Could you check a few things on this model? Use its own coordinates, in mm. A direction names the side the tool comes from. Round coordinates to 2 decimals unless told otherwise and drop trailing zeros. Loops run counter-clockwise (first coordinate to the right, second up) from the corner with the lowest first, then second, coordinate; pieces in that order, holes last. Notation, with made-up numbers: (-5.5, 73) -> (28.5, 73) arc R12 ccw to (28.5, 83) -> close; hole circle Ø5 at (-33.5, 20). An arc over 180 degrees is marked (long way). Put each result on its own line as item: value. Start each with the question number.
1. I need wall thicknesses on line 1 (Y direction, x = 0.75, z = -17); line 2 (Z direction, x = 2.35, y = 11.95); line 3 (Y direction, x = 1.6, z = -8). Which ranges of each line are inside material? Lowest first, please. Write a range as [from, to].
2. Imagine slicing it at A-A, the plane y = 25.81. Please give me the cut outline in (x, z).
3. I'm going to push a flat-ended pin straight in: P1, Ø1.5, axis at x = 1, y = 62, coming from the +Z side. Where does the tip first touch, or does it pass through?
4. Which directions (+Z, -Z, +X, -X, +Y, -Y) give clear straight access to the entire face, cutting with the end or side of a thin tool? Please do faces 1 (the cylindrical face through (2, 22, -31)), 2 (the flat face through (2, 12, -29.15)), 3 (the flat face through (2, 55, -2)).
5. If we mould it in two halves opening along Y, with no side actions, what happens to faces 4 (the flat face through (2, 49, -22)), 5 (the cylindrical face through (1.57, 65.92, -7.36)), 6 (the cylindrical face through (1.568, 43.931, -8.462)), 7 (the cylindrical face through (1.612, 39.854, -1.765))? For each: pulls with the +Y half, pulls with the -Y half, needs draft (parallel to the pull), parting line crosses it, or undercut.
6. Imagine slicing it at D-D, the plane x = 2.1. Count the separate pieces of the cut face and the enclosed holes in it, and give its area (3 significant figures).
7. Imagine slicing it at B-B, the plane z = -7. Please give me the cut outline in (x, y) (3 decimals), and give its area (3 significant figures).
8. Imagine slicing it at C-C, the plane y = 7. Please give me the cut outline in (x, z), and give its area (3 significant figures).
```python
from build123d import *

# Parameters (mm, degrees)
SKETCH1_R             = 5.075
SKETCH1_R_2           = 1.65
SKETCH1_R_3           = 2.1
SKETCH1_R_4           = 0.8
SKETCH1_W             = 13
SKETCH1_H             = 18
BOSS_EXTRUDE1_DEPTH   = 3.18
SKETCH3_R             = 5.5
CUT_EXTRUDE4_DEPTH    = 78.831812262
FILLET2_R             = 3
CHAMFER2_SIZE         = 1.8
FILLET4_R             = 0.5
M2_TAPPED_HOLE1_D     = 1.6
FILLET9_R             = 1
FILLET11_R            = 5
M3X0_5_TAPPED_HOLE1_D = 2.5


with BuildPart() as part:
    # Sketch1 → Boss-Extrude1 (new body)
    with BuildSketch(Plane(origin=(0, 0, 0), x_dir=(0, 0, -1), z_dir=(1, 0, 0))):
        Polygon((0, 0), (0, 37.775), (2, 39.775), (2, 70.81), (22, 70.81), (22, 23.81), (32.15, 23.81), (32.15, 0), align=None)
        with Locations(Location((7, 32.7, 0), (0, 0, 180))):
            Circle(SKETCH1_R, mode=Mode.SUBTRACT)
        with Locations(Location((7, 64.31, 0), (0, 0, 180))):
            Circle(SKETCH1_R_2, mode=Mode.SUBTRACT)
        with Locations(Location((17, 62.31, 0), (0, 0, 180))):
            Circle(SKETCH1_R_2, mode=Mode.SUBTRACT)
        with Locations(Location((3.15, 5.95, 0), (0, 0, 180))):
            Circle(SKETCH1_R_3, mode=Mode.SUBTRACT)
        with Locations(Location((3.15, 11.95, 0), (0, 0, 180))):
            Circle(SKETCH1_R_3, mode=Mode.SUBTRACT)
        with Locations(Location((10.15, 4.95, 0), (0, 0, 180))):
            Circle(SKETCH1_R_4, mode=Mode.SUBTRACT)
        with Locations(Location((3.15, 16.95, 0), (0, 0, 180))):
            Circle(SKETCH1_R_4, mode=Mode.SUBTRACT)
        with Locations((22.65, 11.81)):
            Rectangle(SKETCH1_W, SKETCH1_H, mode=Mode.SUBTRACT)
    extrude(amount=BOSS_EXTRUDE1_DEPTH)

    # Sketch3 → Cut-Extrude4 (cut, through all)
    with BuildSketch(Plane.ZY):
        with Locations((-11, 48.810865899)):
            Circle(SKETCH3_R)
    extrude(amount=-CUT_EXTRUDE4_DEPTH, mode=Mode.SUBTRACT)

    # Fillet2
    fillet2_edges = [part.edges().sort_by_distance(p)[0] for p in [
        (1.59, 0, 0),
        (1.59, 37.775, 0),
        (1.59, 39.775, -2),
    ]]
    fillet(fillet2_edges, radius=FILLET2_R)

    # Chamfer2
    chamfer2_edges = [part.edges().sort_by_distance(p)[0] for p in [
        (1.59, 70.81, -2),
        (1.59, 70.81, -22),
    ]]
    chamfer(chamfer2_edges, length=CHAMFER2_SIZE)

    # Fillet4
    fillet4_edges = [part.edges().sort_by_distance(p)[0] for p in [
        (1.59, 69.01, -22),
        (1.59, 69.01, -2),
    ]]
    fillet(fillet4_edges, radius=FILLET4_R)

    # M2 Tapped Hole1 (through all)
    with Locations(Plane(origin=(0, 16.95, -3.15), x_dir=(0, 0, -1), z_dir=(-1, 0, 0))):
        with Locations((0, 0), (7, 12)):
            Hole(M2_TAPPED_HOLE1_D / 2)

    # Fillet9
    fillet9_edges = [part.edges().sort_by_distance(p)[0] for p in [
        (1.59, 20.81, -16.15),
        (1.59, 2.81, -16.15),
        (1.59, 2.81, -29.15),
        (1.59, 20.81, -29.15),
    ]]
    fillet(fillet9_edges, radius=FILLET9_R)

    # Fillet11
    fillet11_edges = [part.edges().sort_by_distance(p)[0] for p in [
        (1.59, 23.81, -32.15),
        (1.59, 0, -32.15),
        (1.59, 23.81, -22),
    ]]
    fillet(fillet11_edges, radius=FILLET11_R)

    # M3x0.5 Tapped Hole1 (through all)
    with Locations(Plane(origin=(3.18, 0, 0), x_dir=(0, 0, -1), z_dir=(1, 0, 0))):
        with Locations((7, 23.81), (17, 25.81)):
            Hole(M3X0_5_TAPPED_HOLE1_D / 2)


solid = part.part
```
Entries:
1. line 1: [0, 2.82], [20.8, 24.56], [27.06, 60.66], [63.96, 70.81]
1. line 2: [-32.15, -29.15], [-16.15, -5.25], [-1.05, 0]
1. line 3: [0, 23.06], [24.56, 27.72], [37.68, 44.2], [53.42, 63], [65.62, 70.81]
2. outline: (0, -23) -> (3.18, -23) -> (3.18, -18.25) -> (0, -18.25) -> close; (0, -15.75) -> (3.18, -15.75) -> (3.18, 0) -> (0, 0) -> close
3. P1: z = -2
4. face 1: -Z, +X, -X, +Y
4. face 2: +X, -X
4. face 3: +Z, +X, -X, +Y
5. face 4: needs draft
5. face 5: undercut
5. face 6: undercut
5. face 7: pulls with the +Y half
6. separate pieces: 1
6. enclosed holes: 11
6. area: 1,260 mm^2
7. outline: (0, 0) -> (3.18, 0) -> (3.18, 22.56) -> (0, 22.56) -> close; (0, 25.06) -> (3.18, 25.06) -> (3.18, 27.625) -> (0, 27.625) -> close; (0, 37.775) -> (3.18, 37.775) -> (3.18, 45.036) -> (0, 45.036) -> close; (0, 52.586) -> (3.18, 52.586) -> (3.18, 62.66) -> (0, 62.66) -> close; (0, 65.96) -> (3.18, 65.96) -> (3.18, 70.81) -> (0, 70.81) -> close
7. area: 150 mm^2
8. outline: (0, -32.15) -> (3.18, -32.15) -> (3.18, -29.15) -> (0, -29.15) -> close; (0, -16.15) -> (3.18, -16.15) -> (3.18, -4.97) -> (0, -4.97) -> close; (0, -1.33) -> (3.18, -1.33) -> (3.18, 0) -> (0, 0) -> close
8. area: 49.3 mm^2
